Geometry: final body of the model. Coordinates: model frame, mm. Give positions to 0.01 mm unless a question says otherwise; leave off trailing zeros. Write each loop counter-clockwise with the first axis right and the second up, starting at its lowest first coordinate (ties: lowest second). Pieces come first, ordered by that corner, then holes. Notation, with made-up numbers: M 59,46.25 L 105,46.25 A10 ccw 105,53.25 Z; hole C 12,-35.5 d5. An arc over 180 degrees is marked long. Use one line per item in the form item = value. Start each with the question number.
Item 1: Section query B-B on y = -36.5. Return loops of the section in (x, z), then the cut area to 3 significant figures.
Item 2: Section query C-C on x = -645. Return loops of the section in (y, z), then the cut area to 3 significant figures.
Item 3: Section query A-A on z = 333. Return loops of the section in (x, y).
Item 4: Contact query for flat-ended pins moving along their axis: P1, Ø5, axis at x = -720.5, y = -12, coming from the +Z side; P2, Ø21, axis at x = -889, z = 1048, coming from the -Y side; P3, Ø1, axis at y = -68.5, z = 808.5, coming from the +X side. Output: stop coordinate, or through.
Item 5: Material intervals for line 1 along X through (y, z) = (-29.5, 672.5); line 2 along Z through (x, y) = (-248.5, -45.5); line 3 along Y through (x, z) = (-870, 1570), sorted ascending. Write a range as from..to.
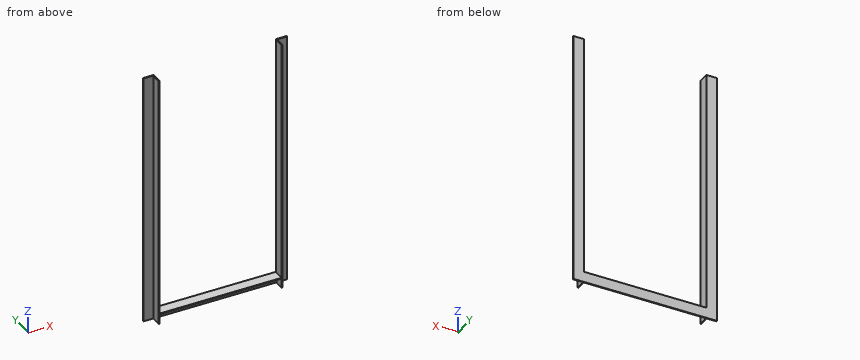
from build123d import *

# Parameters (mm, degrees)
F1_DEPTH = 1828.8
F3_DEPTH = 431.8


with BuildPart() as f1:
    # F0 (on Top) → F1 (new body)
    with BuildSketch(Plane.XY):
        Polygon((0, 0), (0, -76.2), (6.35, -76.2), (6.35, -6.35), (76.2, -6.35), (76.2, 0), align=None)
    extrude(amount=F1_DEPTH)

    # F2 (on face) → F3 (join)
    with BuildSketch(Plane(origin=(0, 0, 0), x_dir=(0, -1, 0), z_dir=(-1, 0, 0))):
        Polygon((0, 76.2), (0, 0), (6.35, 0), (6.35, 69.85), (76.2, 69.85), (76.2, 76.2), align=None)
    extrude(amount=F3_DEPTH)

    # F4: F1 across face


with BuildPart() as f1_1:
    add(f1.part)
    add(f1.part.mirror(Plane(origin=(-431.8, -21.396739, 54.803261), x_dir=(0, -1, 0), z_dir=(-1, 0, 0))))


solid = f1_1.part
Answer sheet:
q1.outline = M -869.95,0 L -863.6,0 L -863.6,69.85 L 0,69.85 L 0,0 L 6.35,0 L 6.35,1828.8 L 0,1828.8 L 0,76.2 L -863.6,76.2 L -863.6,1828.8 L -869.95,1828.8 Z
q1.area = 28,700 mm2
q2.outline = M -76.2,69.85 L -6.35,69.85 L -6.35,0 L 0,0 L 0,76.2 L -76.2,76.2 Z
q2.area = 927 mm2
q3.outline = M -939.8,-6.35 L -869.95,-6.35 L -869.95,-76.2 L -863.6,-76.2 L -863.6,0 L -939.8,0 Z; M 0,-76.2 L 6.35,-76.2 L 6.35,-6.35 L 76.2,-6.35 L 76.2,0 L 0,0 Z
q4.P1 = 76.2
q4.P2 = -6.35
q4.P3 = 6.35
q5.line_1 = -869.95..-863.6, 0..6.35
q5.line_2 = 69.85..76.2
q5.line_3 = -6.35..0
